Autodesk Inventor part; units mm, degrees
ref_plane "YZ Plane" through (0, 0, 0) normal (1, 0, 0) x (0, 1, 0)
ref_plane "XZ Plane" through (0, 0, 0) normal (0, 1, 0) x (-1, 0, 0)
ref_plane "XY Plane" through (0, 0, 0) normal (0, 0, 1) x (1, 0, 0)
sketch "Sketch1" plane through (0, 0, 0) normal (0, 1, 0) x (-1, 0, 0)
  line L0 (0, 0) -> (10, 0)
  line L1 (10, 0) -> (10, -10)
  line L2 (10, -10) -> (0, -10)
  line L3 (0, -10) -> (0, 0)
  line L4 (10, 0) -> (0, -10) construction
  line L5 (10, -10) -> (0, 0) construction
  line L6 (2, -2) -> (8, -2)
  line L7 (8, -2) -> (8, -8)
  line L8 (8, -8) -> (2, -8)
  line L9 (2, -8) -> (2, -2)
  line L10 (2, -2) -> (8, -8) construction
  line L11 (8, -2) -> (2, -8) construction
  point P0 (5, -5)
  dimension "d0" = 10
  dimension "d4" = 6
  dimension "d5" = 6
extrude "Extrusion1" add sketch "Sketch1" along normal blind 30
sketch "Sketch2" plane through (-10, 0, -10) normal (-1, 0, 0) x (0, 0, 1)
  line L0 (0, 30) -> (10, 30) construction
  line L1 (10, 0) -> (0, 0)
  line L2 (10, 0) -> (0, 0) construction
  line L3 (0, 0) -> (0, 7)
  line L4 (0, 7) -> (10, 7)
  line L5 (10, 7) -> (10, 0)
  line L6 (0, 0) -> (0, 30) construction
  line L7 (10, 0) -> (10, 30) construction
  dimension "d8" = 7
  dimension "d9" = 10
extrude "Extrusion2" add sketch "Sketch2" along normal blind 69
chamfer "Chamfer1" distance 20 distance2 38.75 1 edges at (-10, 7, -5) measured on face at (-10, 14.6667, -6.6667)
sketch "Sketch3" plane through (0, 0, 0) normal (0, 0, 1) x (1, 0, 0)
  line L0 (-48.75, 7) -> (-79, 7) construction
  line L1 (-10, 27) -> (-10, 30) construction
  line L2 (-9.9219, 6.8486) -> (-33.7809, 6.8486)
  line L3 (-33.7809, 6.8486) -> (-9.9219, 19.163)
  line L4 (-9.9219, 19.163) -> (-9.9219, 6.8486)
  line L5 (-48.75, 7) -> (-10, 27)
  point P0 (0, 0)
  dimension "d21" = 7
extrude "Extrusion3" cut sketch "Sketch3" against normal through all
sketch "Sketch6" plane through (0, 0, 0) normal (0, -1, 0) x (1, 0, 0)
  line L0 (-79, -10) -> (-79, 0) construction
  line L1 (-79, -5) -> (0, -5) construction
  line L2 (0, 0) -> (0, -10) construction
  line L3 (-24.2304, -1.5) -> (-79, -1.5)
  line L4 (-79, -1.5) -> (-79, -8.5)
  line L5 (-79, -8.5) -> (-24.2304, -8.5)
  line L6 (-24.2304, -8.5) -> (-24.2304, -1.5) construction
  line L7 (-24.2304, -1.5) -> (-79, -8.5) construction
  line L8 (-79, -1.5) -> (-24.2304, -8.5) construction
  line L9 (-24.2304, -8.5) -> (0, -8.5) construction
  line L10 (-24.2304, -1.5) -> (0, -1.5) construction
  line L11 (-24.2304, -8.5) -> (-10, -10)
  line L12 (0, -10) -> (-10, -10) construction
  line L13 (-24.2304, -1.5) -> (-10, 0)
  line L14 (-10, 0) -> (0, 0) construction
  line L15 (-10, -10) -> (-10, -18.6026)
  line L16 (-10, -18.6026) -> (-95.3433, -18.6026)
  line L17 (-95.3433, -18.6026) -> (-95.3433, 10.4)
  line L18 (-95.3433, 10.4) -> (-10, 10.4)
  line L19 (-10, 10.4) -> (-10, 0)
  point P0 (-51.6152, -5)
  dimension "d22" = 7
extrude "Extrusion5" cut sketch "Sketch6" against normal through all
hole "Hole1" at (-79, 3.5, -5) direction (1, 0, 0) diameter 4 depth 5
fillet "Fillet1" radius 1 5 edges at (-33.7809, 6.8486, -5) (-9.9219, 6.8486, -5) (-9.9219, 19.163, -5) (-48.75, 7, -5) (-10, 27, -5)
properties part number "foot_1_2_small"
Check sheet for the modelled part. Datum: model origin and axes. Units: mm. A direction names the side the tool comes from. Give positions to 0.01 mm unless a question says otherwise; leave off trailing zeros. Loops run counter-clockwise (first coordinate to the right, second up) from the corner with the lowest first, then second, coordinate; pieces in that order, holes last. Notation, with made-up numbers: M -23,-9 L 0,-9 A21 cw 0,15 Z; hole C 25.25,-5.5 d11. An arc over 180 degrees is marked long. Use a Markdown table: item, result. Add a question column.
Q1. Scan lines: line 1 along Y through (x, z) = (-76.4, -5); line 2 along X through (y, z) = (5.5, -3.5); line 3 along Z through (x, y) = (-77.8, 3.5). Record each from-to range of solid material in increasing order. Write a range as [from, to].
Q2. Go/stop test with flat-tipped pins: pin 1 (5.5 mm diameter, centred on x = -64, z = -4.5, fed in from +Y); pin 2 (6 mm diameter, centred on x = -42.5, z = -5.5, fed in from +Y); pin 3 (5 mm diameter, centred on y = 14.5, z = -2.5, fed in from -X). Record where each tip stops, or that it passes through.
Q3. Sectioned sample at D-D, the plane x = -21.5. Record the cut outline in (y, z).
Q4. Sectioned sample at B-B, the plane y = 16.5. Record the cut outline in (x, z), then the cut area to 3 significant figures.
Q5. Tool access check on faces 1 (the flat face through (-5, 15, -2)), 2 (the flat face through (-10, 29, -5)), 3 (the flat face through (-46, 5, -8.5)). Record the directions out of +Z, -Z, +X, -X, +Y, -Y that give a thin tool (end or side, any length) a straight path to the whole face; none if there is none.
Q6. Sectioned sample at C-C, the plane y = 3.5. Record the cut outline in (x, z), then the cut area to 3 significant figures.
Q7. Sectioned sample at A-A, the plane z = -5. Record the cut outline in (x, y).
Q8. Mould release check, pull along X, two halves, no side actions. Record for faces 4 (the flat face through (-9.922, 13, -5)), 5 (the flat face through (-8, 15, -5)), 6 (the flat face through (-17.21, 19.58, -0.76)), 7 (the flat face through (-4.9, 30, -1.6)): pulls with the +X half, pulls with the -X half, needs draft (parallel to the pull), parting line crosses it, or undercut.
Verdict:
| question | item | result |
|---|---|---|
| 1 | line 1 | [0, 1.5], [5.5, 7] |
| 1 | line 2 | [-79, -8], [-2, 0] |
| 1 | line 3 | [-8.5, -7], [-3, -1.5] |
| 2 | pin 1 | y = 7 |
| 2 | pin 2 | y = 11.77 |
| 2 | pin 3 | x = -39.06 |
| 3 | outline | M 0,-8.79 L 6.85,-8.79 L 6.85,-1.21 L 0,-1.21 Z; M 13.19,-8.79 L 21.06,-8.79 L 21.06,-1.21 L 13.19,-1.21 Z |
| 4 | outline | M -30.34,-8.5 L -24.23,-8.5 L -15.08,-9.46 L -15.08,-0.54 L -24.23,-1.5 L -30.34,-1.5 Z; M -9.92,-10 L 0,-10 L 0,0 L -9.92,0 Z; hole M -8,-8 L -2,-8 L -2,-2 L -8,-2 Z |
| 4 | area | 179 mm^2 |
| 5 | face 1 | +Y, -Y |
| 5 | face 2 | +Z, -Z, -X, +Y |
| 5 | face 3 | -Z, -X, +Y, -Y |
| 6 | outline | M -79,-8.5 L -24.23,-8.5 L -10,-10 L 0,-10 L 0,0 L -10,0 L -24.23,-1.5 L -79,-1.5 L -79,-3 L -74,-3 L -74,-7 L -79,-7 Z; hole M -8,-8 L -2,-8 L -2,-2 L -8,-2 Z |
| 6 | area | 548 mm^2 |
| 7 | outline | M -79,0 L -8,0 L -8,30 L -10,30 L -10,27.61 A1 cw -10.54,26.72 L -48.53,7.11 A1 cw -48.99,7 L -79,7 L -79,5.5 L -74,5.5 L -74,1.5 L -79,1.5 Z; M -2,0 L 0,0 L 0,30 L -2,30 Z; hole M -30.12,8.74 A1 ccw -29.66,6.85 L -10.92,6.85 A1 ccw -9.92,7.85 L -9.92,17.52 A1 ccw -11.38,18.41 Z |
| 8 | face 4 | undercut |
| 8 | face 5 | undercut |
| 8 | face 6 | pulls with the -X half |
| 8 | face 7 | needs draft |
